Check sheet for the modelled part. Datum: model origin and axes. Units: mm. A direction names the side the tool comes from. Coordinates: 2 decimals unless noted, no trailing zeros. Order: outer loops, then holes, each group sorted by start corner. A loop starts at its lowest first (then second) coordinate and runs counter-clockwise, first axis right, second up.
from build123d import *

# Parameters (mm, degrees)
SKETCH1_W           = 20
SKETCH1_H           = 6
BOSS_EXTRUDE1_DEPTH = 5
CUT_EXTRUDE1_START  = 5
SKETCH1_4_R         = 2.5
SKETCH1_4_R_2       = 2.175
CUT_EXTRUDE1_DEPTH  = 3
CUT_EXTRUDE2_START  = 2
SKETCH1_5_R         = 2.175
CUT_EXTRUDE2_DEPTH  = 5
LPATTERN1_COUNT     = 3
LPATTERN1_PITCH     = 6.5


with BuildPart() as part:
    # Sketch1 → Boss-Extrude1 (new, symmetric)
    with BuildSketch(Plane(origin=(0, 0, 0), x_dir=(1, 0, 0), z_dir=(0, 1, 0))):
        with Locations((0, 3)):
            Rectangle(SKETCH1_W, SKETCH1_H)
    extrude(amount=BOSS_EXTRUDE1_DEPTH, both=True)

    # Sketch1<4> → Cut-Extrude1 (cut)
    # profile 1 of 2: a face of its own
    with BuildSketch(Plane(origin=(0, 0, 0), x_dir=(1, 0, 0), z_dir=(0, 1, 0)).offset(CUT_EXTRUDE1_START)):
        with Locations(Location((-6.516339464, 2.853050679, 0), (0, 0, 270))):
            Circle(SKETCH1_4_R)
        with Locations((-6.516339464, 2.853050679)):
            Circle(SKETCH1_4_R_2, mode=Mode.SUBTRACT)
    # profile 2 of 2: a face of its own
    with BuildSketch(Plane(origin=(0, 0, 0), x_dir=(1, 0, 0), z_dir=(0, 1, 0)).offset(CUT_EXTRUDE1_START)):
        with Locations((-6.516339464, 2.853050679)):
            Circle(SKETCH1_4_R_2)
    cut_extrude1 = extrude(amount=-CUT_EXTRUDE1_DEPTH, mode=Mode.SUBTRACT)

    # Sketch1<5> → Cut-Extrude2 (cut)
    with BuildSketch(Plane(origin=(0, 0, 0), x_dir=(1, 0, 0), z_dir=(0, 1, 0)).offset(CUT_EXTRUDE2_START)):
        with Locations(Location((-6.516339464, 2.853050679, 0), (0, 0, 270))):
            Circle(SKETCH1_5_R)
    cut_extrude2 = extrude(amount=-CUT_EXTRUDE2_DEPTH, mode=Mode.SUBTRACT)

    # LPattern1: Cut-Extrude1, Cut-Extrude2 ×3
    with Locations(*[(i * LPATTERN1_PITCH, 0, 0) for i in range(1, LPATTERN1_COUNT)]):
        add(cut_extrude1, mode=Mode.SUBTRACT)
        add(cut_extrude2, mode=Mode.SUBTRACT)


solid = part.part
(1) Cross-section at A-A (y = -2.75). Enter the section's corners in (x, z) (3 decimals), and give its area (3 significant figures).
Filled in:
outline: (-10, -6) - (10, -6) - (10, 0) - (-10, 0) - close; hole circle Ø4.35 at (-6.516, -2.853); hole circle Ø4.35 at (-0.016, -2.853); hole circle Ø4.35 at (6.484, -2.853)
area: 75.4 mm2
(2) Go/stop test with a flat-tipped pin: P1, Ø3.5, axis at x = -0.02, z = -2.85, coming from the +Y side. Record where the tip stops, or that it passes through.
Filled in:
P1: stops at y = -3
(3) Cross-section at C-C (z = -2.1). Enter the section's corners in (x, y), and give its area (3 significant figures).
Filled in:
outline: (-10, -5) - (10, -5) - (10, 5) - (8.87, 5) - (8.87, 2) - (8.52, 2) - (8.52, -3) - (4.44, -3) - (4.44, 2) - (4.1, 2) - (4.1, 5) - (2.37, 5) - (2.37, 2) - (2.02, 2) - (2.02, -3) - (-2.06, -3) - (-2.06, 2) - (-2.4, 2) - (-2.4, 5) - (-4.13, 5) - (-4.13, 2) - (-4.48, 2) - (-4.48, -3) - (-8.56, -3) - (-8.56, 2) - (-8.9, 2) - (-8.9, 5) - (-10, 5) - close
area: 95.9 mm2
(4) Thickness scan on probe 1 along X at (y, z) = (-2.25, -2.4); probe 2 along Y at (x, z) = (-7, -1); probe 3 along X at (y, z) = (-1.5, -1.25). Record the ranges inside material, lowest first.
Filled in:
probe 1: x = -10 to -8.64, -4.39 to -2.14, 2.11 to 4.36, 8.61 to 10
probe 2: y = -5 to -3
probe 3: x = -10 to -7.99, -5.05 to -1.49, 1.45 to 5.01, 7.95 to 10
(5) Release check for a two-part mould opening along Z. For faces 1 (the cylindrical face through (-5.05, -0.46, -4.46)), 2 (the flat face through (-2.4, 5, -4.4)), 3 (the cylindrical face through (-0.97, 3.52, -0.54)), 4 (the flat face through (0, 0, -6)) record: +Z half, -Z half, draft (parallel to the pull), parting line (faces both ways), or undercut.
Filled in:
face 1: undercut
face 2: draft
face 3: undercut
face 4: -Z half
(6) Cross-section at D-D (y = 4.25). Enter the section's corners in (x, z), and give its area (3 significant figures).
Filled in:
outline: (-10, -6) - (10, -6) - (10, 0) - (-10, 0) - close; hole circle Ø5 at (-6.52, -2.85); hole circle Ø5 at (-0.02, -2.85); hole circle Ø5 at (6.48, -2.85)
area: 61.1 mm2
(7) Tool access check on faces 5 (the flat face through (10, 0, -3)), 6 (the cylindrical face through (7.235, 3.521, -0.468)). Record the directions out of +Z, -Z, +X, -X, +Y, -Y that give a thin tool (end or side, any length) a straight path to the whole face; none if there is none.
Filled in:
face 5: +Z, -Z, +X, +Y, -Y
face 6: +Y
(8) Cross-section at B-B (x = -0.25). Enter the section's corners in (y, z), and give its area (3 significant figures).
Filled in:
outline: (-5, -6) - (5, -6) - (5, -5.34) - (2, -5.34) - (2, -5.02) - (-3, -5.02) - (-3, -0.69) - (2, -0.69) - (2, -0.36) - (5, -0.36) - (5, 0) - (-5, 0) - close
area: 23.4 mm2
